Autodesk Fusion 360 part; units mm, degrees
sketch "Sketch1" plane through (0, 0, 0) normal (0, 1, 0) x (1, 0, 0)
  line L0 (-37, 0) -> (37, 0)
  line L1 (37, 0) -> (37, 22)
  line L2 (37, 22) -> (25, 22)
  line L3 (25, 22) -> (25, 12)
  line L4 (25, 12) -> (-25, 12)
  line L5 (-25, 12) -> (-25, 22)
  line L6 (-25, 22) -> (-37, 22)
  line L7 (-37, 22) -> (-37, 0)
  circle A0 centre (0, -34) radius 15
  circle A1 centre (0, -34) radius 30
  line L8 (-30, 0) -> (-30, -34)
  line L9 (30, 0) -> (30, -34)
  circle A2 centre (65, -28) radius 7
  circle A3 centre (65, -28) radius 14
  line L10 (37, 22) -> (75.1738, -18.3827)
  arc A4 (65.7795, -41.9783) -> (17.0566, -58.6794) centre (71.069, -136.8309) ccw
  dimension "d1" = 25
  dimension "d2" = 25
  dimension "d3" = 37
  dimension "d4" = 37
  dimension "d5" = 22
  dimension "d6" = 22
  dimension "d7" = 12
  dimension "d8" = 12
  dimension "d9" = 30
  dimension "d10" = 34
  dimension "d11" = 37
  dimension "d12" = 60
  dimension "d13" = 14
  dimension "d14" = 28
  dimension "d15" = 65
  dimension "d16" = 28
  dimension "d17" = 190
extrude "Extrude1" add sketch "Sketch1" against normal blind 26 contours L0 L1 L2 L3 L4 L5 L6 L7
extrude "Extrude2" add sketch "Sketch1" against normal blind 20 contours L0 A1 L8 L9 | A1
extrude "Extrude3" add sketch "Sketch1" against normal blind 14 contours L0 L1 A1 L9 A3 L10 A4 | A3
mirror "Mirror1" about plane through (0, 0, 0) normal (1, 0, 0) of "Extrude3"
equation "d1 = ( 50 / 2 ) * 1 mm"
equation "d2 = d1"
equation "d3 = d1 + 12 mm"
equation "d4 = d3"
equation "d7 = d6 - 10 mm"
equation "d8 = d7"
equation "d11 = d3"
equation "d14 = ( 14 * 2 ) * 1 mm"
equation "d15 = ( 130 / 2 ) * 1 mm"
equation "d16 = 50 mm - 22 mm"
equation "d17 = ( 95 * 2 ) * 1 mm"
Part model, mm, in its own coordinate system. A direction names the side the tool comes from. Coordinates: 2 decimals unless noted, no trailing zeros. Write each loop counter-clockwise with the first axis right and the second up, starting at its lowest first coordinate (ties: lowest second). Pieces come first, ordered by that corner, then holes.
Item 1: Slice it at C-C (z = 26.5). Write the cut outline in (x, y).
Item 2: Slice it at B-B (x = 0). Write the cut outline in (y, z), and give its area (3 significant figures).
Item 3: Probe line 1 (X direction, y = -11.75, z = 34); line 2 (X direction, y = -6, z = 28); line 3 (Y direction, x = 46, z = -2). List the from-to ranges inside material, lowest first.
Item 4: Pin check, flat tips, straight feed: pin 1 (11 mm diameter, centred on x = 65, z = 28, fed in from -Y); pin 2 (5 mm diameter, centred on y = -18, z = 19.5, fed in from -X); pin 3 (13 mm diameter, centred on y = -21.5, z = -7, fed in from -X); pin 4 (3.5 mm diameter, centred on y = -21.5, z = -9.5, fed in from +X). Stop position of each tip, or through.
Item 5: Slice it at D-D (z = 52). Write the cut outline in (x, y).
Item 6: Slice it at A-A (y = -18.5). Write the cut outline in (x, z), and give its area (3 significant figures).
Item 7: Mould opens along X. For faces 1 (the face through (-25, -13, -17)), 2 (the face through (-0.66, -12.082, 63.993)), 3 (the face through (25, -13, -17)), 4 (the face through (-48, -14, 18)) say: released by +X, released by -X, zero draft, split by the parting line, or undercut.
Item 8: Which spindle directions (+Z, -Z, +X, -X, +Y, -Y) get a long thin tool onto all of the face, cutting with end or side? Do faces 5 (the face through (0, -20, 17)), 6 (the face through (30, -17, 17)), 7 (the face through (-30, -17, 17)). Say none if no direction does.
Results found:
1. outline: (-78.92, -14) - (-71.84, -14) - (-71.84, 0) - (-78.92, 0) - close; (-58.16, -14) - (-30, -14) - (-30, -20) - (-12.99, -20) - (-12.99, 0) - (-58.16, 0) - close; (12.99, -20) - (30, -20) - (30, -14) - (58.16, -14) - (58.16, 0) - (12.99, 0) - close; (71.84, -14) - (78.92, -14) - (78.92, 0) - (71.84, 0) - close
2. outline: (-26, -12) - (0, -12) - (0, 19) - (-20, 19) - (-20, 0) - (-26, 0) - close; (-20, 49) - (0, 49) - (0, 64) - (-20, 64) - close
2. area: 992 mm2
3. line 1: x = -77.65 to -68.61, -61.39 to -15, 15 to 61.39, 68.61 to 77.65
3. line 2: x = -79 to -72, -58 to -13.75, 13.75 to 58, 72 to 79
3. line 3: y = -14 to 0
4. pin 1: passes through
4. pin 2: stops at x = -30
4. pin 3: stops at x = -37
4. pin 4: stops at x = 37
5. outline: (-28.31, -14) - (-24, -14) - (-24, -20) - (24, -20) - (24, -14) - (28.31, -14) - (28.31, 0) - (-28.31, 0) - close
6. outline: (-37, -22) - (-25, -22) - (-25, -12) - (25, -12) - (25, -22) - (37, -22) - (37, 0) - (30, 0) - (30, 34) arc R30 ccw to (-30, 34) - (-30, 0) - (-37, 0) - close; hole circle Ø30 at (0, 34)
6. area: 3,870 mm2
7. face 1: undercut
7. face 2: split by the parting line
7. face 3: undercut
7. face 4: zero draft
8. face 5: +Z, +X, -X, -Y
8. face 6: +Z, +X, -Y
8. face 7: +Z, -X, -Y
